The model under review builds one solid part; all positions refer to its coordinate system, in mm. Face numbers are marked on the shaded views. A direction names the side the tool comes from. Give positions to 0.01 mm unless a question says otherwise; leave off trailing zeros. Order: outer loops, then holes, each group sorted by start corner. A loop starts at its lowest first (then second) coordinate and runs counter-clockwise, first axis right, second up. Notation, with made-up numbers: (79, 86.25) - (126, 86.25) arc R14 cw to (126, 92.25) - close; hole circle Ø2 at (66.25, -8.5). An arc over 180 degrees is marked (long way). Answer as CSV lines item,"result". Start each with the question number.
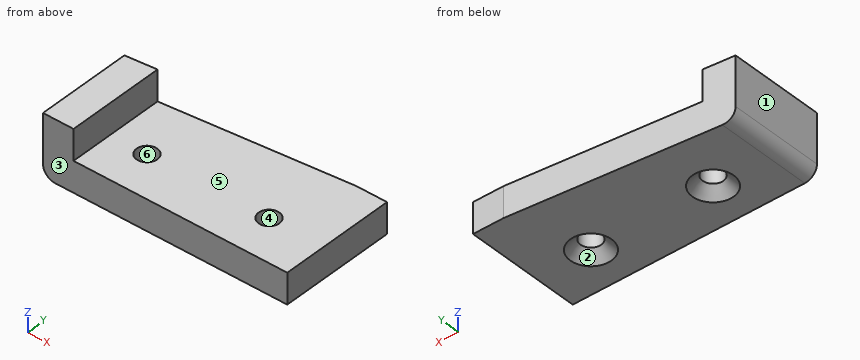
from build123d import *

# Parameters (mm, degrees)
F1_DEPTH       = 19
F3_DEPTH       = 25
F4_D           = 3.4
F4_CSINK_D     = 6.72
F4_CSINK_ANGLE = 90
F5_R           = 2


with BuildPart() as f1:
    # F0 (on Front) → F1 (new body)
    with BuildSketch(Plane.XZ):
        Polygon((-40, 0), (0, 0), (0, 5), (-35, 5), (-35, 10), (-40, 10), align=None)
    extrude(amount=F1_DEPTH)

    # F2 (on face) → F3 (cut)
    with BuildSketch(Plane(origin=(0, 0, 0), x_dir=(1, 0, 0), z_dir=(0, 0, -1))):
        Polygon((-5, 0), (-40, 3.5), (-40, 0), align=None)
    extrude(amount=-F3_DEPTH, mode=Mode.SUBTRACT)

    # F4 (through all)
    with Locations(Plane(origin=(0, 0, 0), x_dir=(1, 0, 0), z_dir=(0, 0, -1))):
        with Locations((-9, 12), (-29, 12)):
            CounterSinkHole(F4_D / 2, F4_CSINK_D / 2, counter_sink_angle=F4_CSINK_ANGLE)

    # F5
    f5_edges = [f1.edges().sort_by_distance(p)[0] for p in [
        (-40, -11.25, 0),
    ]]
    fillet(f5_edges, radius=F5_R)


solid = f1.part
Item 1: Take a section at A-A on x = -29. Write out the cut boundary in (y, z), and give its area (3 significant figures).
Item 2: For line 1 along X through (y, z) = (-12, 2.65); line 2 along X through (y, z) = (-10.75, 4.75); line 3 along Z through (x, y) = (-11, -16.25), list the stretches that pass through material, from the lowest coordinate up.
Item 3: Mouldability with a two-part tool opening along X and no side actions: class the marked faces 1, 2, 3 and 4 as released by +X, released by -X, zero draft, split by the parting line, or undercut.
Item 4: Machinability: for the marked faces 5 and 6, which of the approach directions +Z, -Z, +X, -X, +Y, -Y give a long, thin tool a straight path to every point of the face, cutting with its end or side? Answer none if there is none.
Item 5: Take a section at C-C on y = -12. Write out the cut boundary in (x, z), and give its area (3 significant figures).
Item 6: Clearance check with flat-ended pins moving along their axes: pin 1 (1.5 mm diameter, centred on y = -9.5, z = 7, fed in from +X); pin 2 (1.5 mm diameter, centred on x = -31, y = -2.5, fed in from +Z); pin 3 (4 mm diameter, centred on x = -29, y = -12, fed in from -Z). State where each tip first meets the part, or that it passes through.
Item 7: Take a section at B-B on z = 4.5. Write out the cut boundary in (x, y), and give its area (3 significant figures).
Item 8: Take a section at D-D on x = -9. Write out the cut boundary in (y, z).
Data:
1,outline,"(-19, 0) - (-15.36, 0) - (-13.7, 1.66) - (-13.7, 5) - (-19, 5) - close; (-10.3, 1.66) - (-8.64, 0) - (-2.4, 0) - (-2.4, 5) - (-10.3, 5) - close"
1,area,"63.2 mm^2"
2,line 1,"x = -40 to -30.7, -27.3 to -10.7, -7.3 to 0"
2,line 2,"x = -40 to -30.15, -27.85 to -10.15, -7.85 to 0"
2,line 3,"z = 0 to 5"
3,face 1,"released by -X"
3,face 2,"undercut"
3,face 3,"zero draft"
3,face 4,"undercut"
4,face 5,"+Z, +X, +Y, -Y"
4,face 6,"+Z, -Z"
5,outline,"(-40, 2) arc R2 ccw to (-38, 0) - (-32.36, 0) - (-30.7, 1.66) - (-30.7, 5) - (-35, 5) - (-35, 10) - (-40, 10) - close; (-27.3, 1.66) - (-25.64, 0) - (-12.36, 0) - (-10.7, 1.66) - (-10.7, 5) - (-27.3, 5) - close; (-7.3, 1.66) - (-5.64, 0) - (0, 0) - (0, 5) - (-7.3, 5) - close"
5,area,"185 mm^2"
6,pin 1,"stops at x = -35"
6,pin 2,"stops at z = 5"
6,pin 3,"stops at z = 1.36"
7,outline,"(-40, -19) - (0, -19) - (0, 0) - (-5, 0) - (-40, -3.5) - close; hole circle Ø3.4 at (-29, -12); hole circle Ø3.4 at (-9, -12)"
7,area,"681 mm^2"
8,outline,"(-19, 0) - (-15.36, 0) - (-13.7, 1.66) - (-13.7, 5) - (-19, 5) - close; (-10.3, 1.66) - (-8.64, 0) - (-0.4, 0) - (-0.4, 5) - (-10.3, 5) - close"
